```python
from build123d import *

# Parameters (mm, degrees)
SKETCH_1_R          = 12.5
EXTRUDE_1_DEPTH     = 2
SKETCH_2_R          = 7.5
EXTRUDE_2_DEPTH     = 2
FILLET_1_R          = 1
CUT_EXTRUDE_1_REACH = 20.125
SKETCH_3_R          = 2.6
SKETCH_4_W          = 78.608538246
SKETCH_4_H          = 29.839159416
EXTRUDE_3_DEPTH     = 5


with BuildPart() as part:
    # 草图1 → 凸台-拉伸1 (new body)
    with BuildSketch(Plane(origin=(0, 0, 0), x_dir=(1, 0, 0), z_dir=(0, 1, 0))):
        with Locations(Location((0, 0, 0), (0, 0, 270))):
            Circle(SKETCH_1_R)
    extrude(amount=EXTRUDE_1_DEPTH)

    # 草图2 → 凸台-拉伸2 (add)
    with BuildSketch(Plane(origin=(0, 2, 0), x_dir=(1, 0, 0), z_dir=(0, 1, 0))):
        with Locations(Location((0, 0, 0), (0, 0, 270))):
            Circle(SKETCH_2_R)
    extrude(amount=EXTRUDE_2_DEPTH)

    # 圆角1
    fillet_1_edges = [part.edges().sort_by_distance(p)[0] for p in [
        (0, 2, -7.5),
    ]]
    fillet(fillet_1_edges, radius=FILLET_1_R)

    # 草图3 → 切除-拉伸1 (cut, up to next)
    with BuildSketch(Plane(origin=(0, 4, 0), x_dir=(1, 0, 0), z_dir=(0, 1, 0)), mode=Mode.PRIVATE) as cut_extrude_1_sk1:
        with Locations(Location((0, 0, 0), (0, 0, 270))):
            Circle(SKETCH_3_R)
    cut_extrude_1_tool1 = extrude(cut_extrude_1_sk1.sketch, amount=-CUT_EXTRUDE_1_REACH, mode=Mode.PRIVATE) & part.part
    add(cut_extrude_1_tool1.solids().sort_by_distance((0, 4, 0))[0], mode=Mode.SUBTRACT)

    # 草图4 → 凸台-拉伸3 (add)
    with BuildSketch(Plane(origin=(0, 0, 0), x_dir=(1, 0, 0), z_dir=(0, 1, 0))):
        Rectangle(SKETCH_4_W, SKETCH_4_H)
    extrude(amount=-EXTRUDE_3_DEPTH)


solid = part.part
```
Could you check a few things on this model? Use its own coordinates, in mm. A direction names the side the tool comes from. Give positions to 0.01 mm unless a question says otherwise; leave off trailing zeros. Write each loop counter-clockwise with the first axis right and the second up, starting at its lowest first coordinate (ties: lowest second). Pieces come first, ordered by that corner, then holes. Notation, with made-up numbers: (29, 74) - (75, 74) arc R31 cw to (75, 108) - close; hole circle Ø6 at (-16.5, 65.25). An arc over 180 degrees is marked (long way). One line per item, written item: value. Start each with the question number.
Item 1: Please list where these lines run through material, in increasing order: line 1 (X direction, y = 2.95, z = 0); line 2 (X direction, y = 1.6, z = 0); line 3 (Y direction, x = -13, z = 11.25). Write a range as from..to.
Item 2: Imagine slicing it at A-A, the plane z = -10. List the corners of the cut face in (x, y) for me.
Item 3: I'm going to push flat-ended pins straight in: pin 1 (1.6 mm diameter, centred on x = -1, z = 0.5, fed in from +Y); pin 2 (2 mm diameter, centred on y = 2, z = -6.5, fed in from -X) (3 decimals). Where does each tip first touch, or does it pass through?
Item 4: Imagine slicing it at B-B, the plane x = 0. List the corners of the cut face in (y, z) for me.
Item 5: Imagine slicing it at C-C, the plane z = 0. List the corners of the cut face in (x, y) for me, and give its area (3 significant figures).
Item 6: If we mould it in two halves opening along X, with no side actions, what happens to faces 3 (the face through (-1, -2, 14.92)), 4 (the face through (39.304, -2, 0)), 5 (the face through (0, 0, 0))? For each: +X half, -X half, draft (parallel to the pull), parting line (faces both ways), or undercut.
Item 7: Imagine slicing it at D-D, the plane x = 14. List the corners of the cut face in (y, z) for me, and give its area (3 significant figures).
Item 8: Which directions (+Z, -Z, +X, -X, +Y, -Y) give clear straight access to the entire face, cutting with the end or side of a thin tool? Please do faces 1 (the face through (0.33, 3.493, -7.493)), 2 (the face through (-1, -5, 0)).
Geometry says:
1. line 1: -7.5..-2.6, 2.6..7.5
1. line 2: -12.5..-2.6, 2.6..12.5
1. line 3: -5..0
2. outline: (-39.3, -5) - (39.3, -5) - (39.3, 0) - (7.5, 0) - (7.5, 2) - (-7.5, 2) - (-7.5, 0) - (-39.3, 0) - close
3. pin 1: y = 0
3. pin 2: x = -11.225
4. outline: (-5, -14.92) - (0, -14.92) - (0, -12.5) - (2, -12.5) - (2, -8.5) arc R1 cw to (3, -7.5) - (4, -7.5) - (4, -2.6) - (0, -2.6) - (0, 2.6) - (4, 2.6) - (4, 7.5) - (3, 7.5) arc R1 cw to (2, 8.5) - (2, 12.5) - (0, 12.5) - (0, 14.92) - (-5, 14.92) - close
5. outline: (-39.3, -5) - (39.3, -5) - (39.3, 0) - (12.5, 0) - (12.5, 2) - (8.5, 2) arc R1 cw to (7.5, 3) - (7.5, 4) - (2.6, 4) - (2.6, 0) - (-2.6, 0) - (-2.6, 4) - (-7.5, 4) - (-7.5, 3) arc R1 cw to (-8.5, 2) - (-12.5, 2) - (-12.5, 0) - (-39.3, 0) - close
5. area: 453 mm^2
6. face 3: draft
6. face 4: +X half
6. face 5: undercut
7. outline: (-5, -14.92) - (0, -14.92) - (0, 14.92) - (-5, 14.92) - close
7. area: 149 mm^2
8. face 1: +Y
8. face 2: +Z, -Z, +X, -X, -Y
